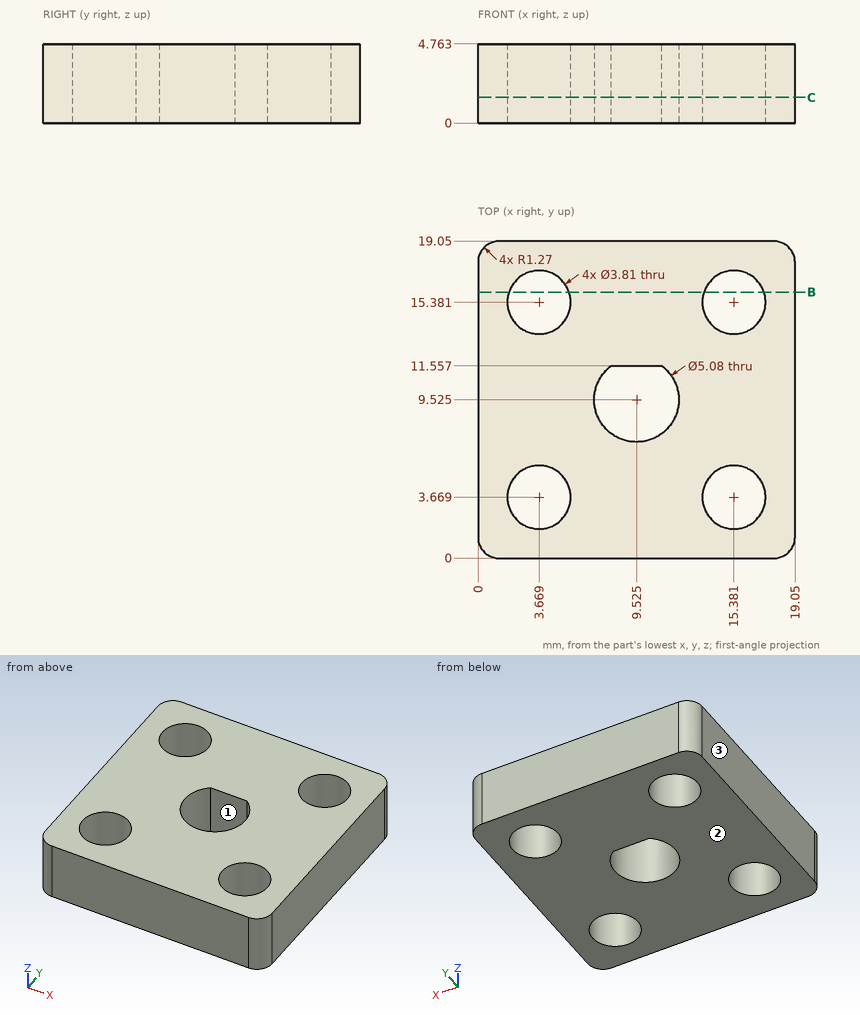
Design review of the part shown in the three views and the two pictorial views. Dimensions are in mm from the part's minimum x, y and z. Give positions to 0.01 mm unless a question says otherwise; leave off trailing zeros. Loops run counter-clockwise (first coordinate to the right, second up) from the corner with the lowest first, then second, coordinate; pieces in that order, holes last. Notation, with made-up numbers: M 14,65 L 69,65 A20 cw 69,84 Z; hole C 45.5,42 d3. An arc over 180 degrees is marked long. Answer as a JSON object with one key per item and string values. Group by question number.
Q1. Add section B-B on y = 16. Give the boundary of the cut face in (x, z).
Q2. Insertion check: P1, Ø4, axis at x = 9.525, y = 9.525, coming from the -Z side. The pin has a flat end and moves straight along its axis. Give the tip position at first contact, or say it passes through.
Q3. Add section C-C on z = 1.55. Give the number of separate pieces and of enclosed holes in the cut face, and give its area (3 significant figures).
Q4. Mouldability with a two-part tool opening along X and no side actions: class the marked faces 1, 2 and 3 as +X half, -X half, draft (parallel to the pull), parting line (faces both ways), or undercut.
Q5. For probe 1 along X at (y, z) = (2.75, 3.7); probe 2 along Y at (x, z) = (14.5, 2.15); probe 3 along Y at (x, z) = (10.25, 3.6), list the stretches that pass through material, from the lowest coordinate up. Write a range as [from, to].
Checked values:
{
 "1": {"outline": "M 0,0 L 1.87,0 L 1.87,4.76 L 0,4.76 Z; M 5.47,0 L 13.58,0 L 13.58,4.76 L 5.47,4.76 Z; M 17.18,0 L 19.05,0 L 19.05,4.76 L 17.18,4.76 Z"},
 "2": {"P1": "through"},
 "3": {"separate pieces": "1", "enclosed holes": "5", "area": "297 mm²"},
 "4": {"face 1": "undercut", "face 2": "draft", "face 3": "-X half"},
 "5": {"probe 1": "[0, 2], [5.34, 13.71], [17.05, 19.05]", "probe 2": "[0, 1.98], [5.36, 13.69], [17.07, 19.05]", "probe 3": "[0, 7.09], [11.56, 19.05]"}
}
